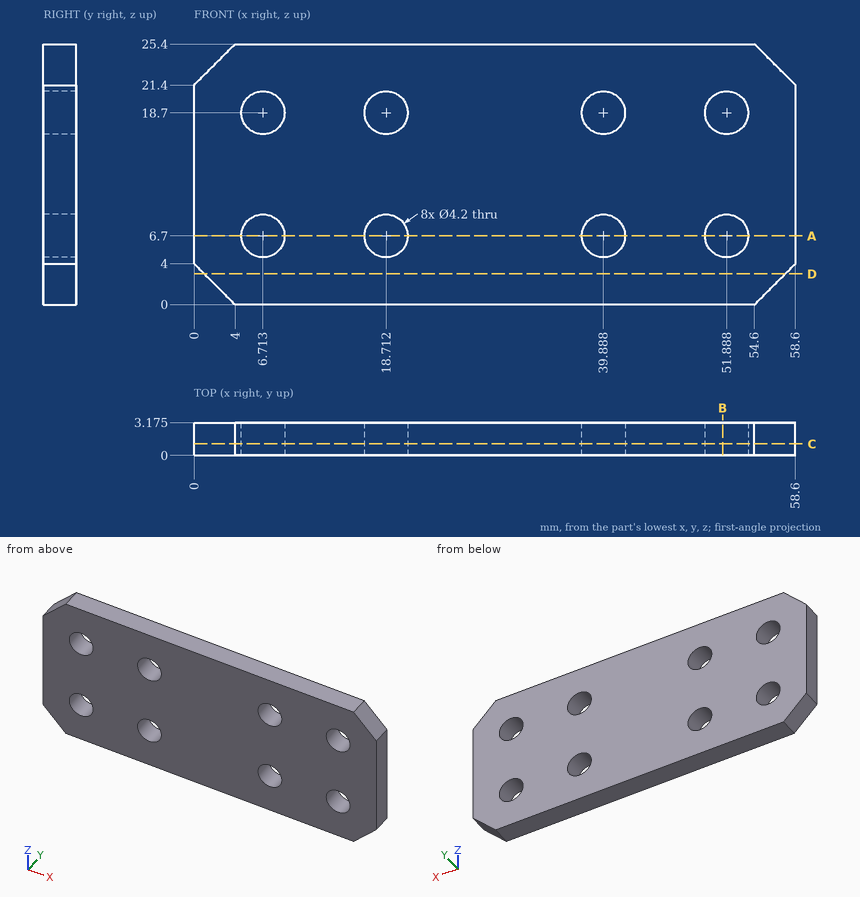
The drawing under review shows one solid part. Ordinate dimensions are in mm from its lowest x, y, z. Round coordinates to 2 decimals unless told otherwise and drop trailing zeros. Write each loop counter-clockwise with the first axis right and the second up, starting at its lowest first coordinate (ties: lowest second). Pieces come first, ordered by that corner, then holes. Notation, with made-up numbers: (-11.75, 43) - (33.25, 43) arc R18 ccw to (33.25, 55) - close; hole circle Ø6 at (-20.75, 80.25). An arc over 180 degrees is marked (long way). Use a Markdown table: item, result. Add a question column.
1. We need section C-C (y = 1.1). Count the separate pieces of the cut face and the enclosed holes in it, then the cut area to 3 significant figures.
2. Wall thickness on probe 1 along Z at (x, y) = (8, 0.3); probe 2 along Z at (x, y) = (7, 2.75); probe 3 along X at (y, z) = (0.85, 8) (1 decimal): over which ranges is each line inside the solid? List them lowest first.
3. We need section B-B (x = 51.5). State the section outline as (y, z) points (1 decimal).
4. We need section D-D (z = 3). State the section outline as (x, y) points (1 decimal), then the cut area to 3 significant figures.
5. We need section A-A (z = 6.7). State the section outline as (x, y) points (1 decimal).
Output:
| question | item | result |
|---|---|---|
| 1 | separate pieces | 1 |
| 1 | enclosed holes | 8 |
| 1 | area | 1,350 mm2 |
| 2 | probe 1 | z = 0 to 5.04, 8.36 to 17.04, 20.36 to 25.4 |
| 2 | probe 2 | z = 0 to 4.62, 8.78 to 16.62, 20.78 to 25.4 |
| 2 | probe 3 | x = 0 to 5.1, 8.4 to 17.1, 20.4 to 38.2, 41.5 to 50.2, 53.5 to 58.6 |
| 3 | outline | (0, 0) - (3.2, 0) - (3.2, 4.6) - (0, 4.6) - close; (0, 8.8) - (3.2, 8.8) - (3.2, 16.6) - (0, 16.6) - close; (0, 20.8) - (3.2, 20.8) - (3.2, 25.4) - (0, 25.4) - close |
| 4 | outline | (1, 0) - (57.6, 0) - (57.6, 3.2) - (1, 3.2) - close |
| 4 | area | 180 mm2 |
| 5 | outline | (0, 0) - (4.6, 0) - (4.6, 3.2) - (0, 3.2) - close; (8.8, 0) - (16.6, 0) - (16.6, 3.2) - (8.8, 3.2) - close; (20.8, 0) - (37.8, 0) - (37.8, 3.2) - (20.8, 3.2) - close; (42, 0) - (49.8, 0) - (49.8, 3.2) - (42, 3.2) - close; (54, 0) - (58.6, 0) - (58.6, 3.2) - (54, 3.2) - close |
